from build123d import *

# Parameters (mm, degrees)
SKETCH1_R           = 40
BOSS_EXTRUDE1_DEPTH = 0.6
SKETCH2_R           = 42.5
BOSS_EXTRUDE2_DEPTH = 4
SKETCH3_R           = 22.5
CUT_EXTRUDE1_DEPTH  = 61.279847379
SKETCH4_R           = 1.2
CUT_EXTRUDE4_DEPTH  = 61.279847379


with BuildPart() as part:
    # Sketch1 → Boss-Extrude1 (new body)
    with BuildSketch(Plane(origin=(0, 0, 0), x_dir=(1, 0, 0), z_dir=(0, 1, 0))):
        with Locations(Location((0, 0, 0), (0, 0, 270))):
            Circle(SKETCH1_R)
    extrude(amount=BOSS_EXTRUDE1_DEPTH)

    # Sketch2 → Boss-Extrude2 (add)
    with BuildSketch(Plane(origin=(0, 0.6, 0), x_dir=(1, 0, 0), z_dir=(0, 1, 0))):
        with Locations(Location((0, 0, 0), (0, 0, 270))):
            Circle(SKETCH2_R)
    extrude(amount=BOSS_EXTRUDE2_DEPTH)

    # Sketch3 → Cut-Extrude1 (cut, through all)
    with BuildSketch(Plane.XZ):
        with Locations(Location((0, 0, 0), (0, 0, 270))):
            Circle(SKETCH3_R)
    extrude(amount=-CUT_EXTRUDE1_DEPTH, mode=Mode.SUBTRACT)

    # Sketch4 → Cut-Extrude4 (cut, through all)
    with BuildSketch(Plane.XZ):
        with Locations(Location((0, 35, 0), (0, 0, 270))):
            Circle(SKETCH4_R)
        with Locations(Location((24.748737342, 24.748737342, 0), (0, 0, 270))):
            Circle(SKETCH4_R)
        with Locations(Location((35, 0, 0), (0, 0, 270))):
            Circle(SKETCH4_R)
        with Locations(Location((24.748737342, -24.748737342, 0), (0, 0, 270))):
            Circle(SKETCH4_R)
        with Locations(Location((0, -35, 0), (0, 0, 270))):
            Circle(SKETCH4_R)
        with Locations(Location((-24.748737342, -24.748737342, 0), (0, 0, 270))):
            Circle(SKETCH4_R)
        with Locations(Location((-35, 0, 0), (0, 0, 270))):
            Circle(SKETCH4_R)
        with Locations(Location((-24.748737342, 24.748737342, 0), (0, 0, 270))):
            Circle(SKETCH4_R)
    extrude(amount=-CUT_EXTRUDE4_DEPTH, mode=Mode.SUBTRACT)


solid = part.part
Input: part model. Units: mm. Frame: model coordinates. A direction names the side the tool comes from. Give positions to 0.01 mm unless a question says otherwise; leave off trailing zeros. Order: outer loops, then holes, each group sorted by start corner. A loop starts at its lowest first (then second) coordinate and runs counter-clockwise, first axis right, second up. Notation, with made-up numbers: (44.5, 74.25) -> (70.5, 74.25) arc R18 cw to (70.5, 97.25) -> close; hole circle Ø6 at (18.25, 75.25). An arc over 180 degrees is marked (long way). Use one line per item in the form item = value.
1) Section D-D, the plane z = -14. Return loops of the section in (x, y), and give its area (3 significant figures).
Response values:
outline = (-40.13, 0.6) -> (-37.47, 0.6) -> (-37.47, 0) -> (-17.61, 0) -> (-17.61, 4.6) -> (-40.13, 4.6) -> close; (17.61, 0) -> (37.47, 0) -> (37.47, 0.6) -> (40.13, 0.6) -> (40.13, 4.6) -> (17.61, 4.6) -> close
area = 204 mm^2
2) First-contact query: pin 1 Ø2 at (y, z) = (1.5, -21.5) entering from +X; pin 2 Ø1.5 at (y, z) = (3, -13.5) entering from -X; pin 3 Ø1 at (y, z) = (0.5, -23.5) entering from +X; pin 4 Ø2 at (x, z) = (-24.75, 24.75) entering from +Y. Flat tips, straight axial feed; report the tip coordinate or a pass-through.
Response values:
pin_1 = 37.23
pin_2 = -40.54
pin_3 = 35.73
pin_4 = through
3) Line query: probe 1 along X at (y, z) = (1.5, 0); probe 2 along X at (y, z) = (2.45, 35); probe 3 along Z at (x, y) = (-24, 2.85). Output: solid intervals per line, ascending.
Response values:
probe_1 = -42.5 to -36.2, -33.8 to -22.5, 22.5 to 33.8, 36.2 to 42.5
probe_2 = -24.11 to -1.2, 1.2 to 24.11
probe_3 = -35.07 to -25.69, -23.81 to 23.81, 25.69 to 35.07
4) Section A-A, the plane x = 0. Return loops of the section in (y, z).
Response values:
outline = (0, -40) -> (0.6, -40) -> (0.6, -42.5) -> (4.6, -42.5) -> (4.6, -36.2) -> (0, -36.2) -> close; (0, -33.8) -> (4.6, -33.8) -> (4.6, -22.5) -> (0, -22.5) -> close; (0, 22.5) -> (4.6, 22.5) -> (4.6, 33.8) -> (0, 33.8) -> close; (0, 36.2) -> (4.6, 36.2) -> (4.6, 42.5) -> (0.6, 42.5) -> (0.6, 40) -> (0, 40) -> close
5) Reachability of faces 5 (the flat face through (-28, 0.6, -29)), 6 (the cylindrical face through (25.76, 2.27, 24.1)) from +Z, -Z, +X, -X, +Y, -Y: full face, straight path, thin tool, end or side. Return the list, or none.
Response values:
face_5 = -Y
face_6 = +Y, -Y
6) Section B-B, the plane y = 2.65. Count the separate pieces of the cut face and the enclosed holes in it, and give its area (3 significant figures).
Response values:
separate_pieces = 1
enclosed_holes = 9
area = 4,050 mm^2
7) Mould query, pull axis X, two halves, no side actions, for faces 1 (the cylindrical face through (-8.618, 2.268, -20.784)), 2 (the flat face through (-17, 0, 17)), 3 (the cylindrical face through (-25.861, 2.572, -33.727)), 4 (the cylindrical face through (-24.4, 2.3, 23.6)). Classes: pulls with the +X half, pulls with the -X half, needs draft (parallel to the pull), parting line crosses it, or undercut.
Response values:
face_1 = undercut
face_2 = needs draft
face_3 = parting line crosses it
face_4 = undercut
8) Section C-C, the plane x = 35. Return loops of the section in (y, z), and give its area (3 significant figures).
Response values:
outline = (0, -19.36) -> (0.6, -19.36) -> (0.6, -24.11) -> (4.6, -24.11) -> (4.6, -1.2) -> (0, -1.2) -> close; (0, 1.2) -> (4.6, 1.2) -> (4.6, 24.11) -> (0.6, 24.11) -> (0.6, 19.36) -> (0, 19.36) -> close
area = 205 mm^2
